Work out the finished part from the listing and answer in its coordinate system (mm). A direction names the side the tool comes from. Coordinates: 2 decimals unless noted, no trailing zeros. Order: outer loops, then holes, each group sorted by start corner. A loop starts at its lowest first (then second) coordinate and runs counter-clockwise, first axis right, second up.
```python
from build123d import *

# Parameters (mm, degrees)
EXTRUDE_1_DEPTH     = 25
EXTRUDE_3_DEPTH     = 4
EXTRUDE_4_DEPTH     = 4
EXTRUDE_5_DEPTH     = 4
EXTRUDE_6_DEPTH     = 4
EXTRUDE_7_DEPTH     = 7
SKETCH_7_W          = 23
SKETCH_7_H          = 20
EXTRUDE_8_DEPTH     = 8.5
SKETCH_8_W          = 16.231712275
SKETCH_8_H          = 15.860541866
EXTRUDE_9_DEPTH     = 3
FILLET_1_R          = 3
FILLET_2_R          = 1
SKETCH_9_R          = 10.42057087
CUT_EXTRUDE_1_DEPTH = 1
SKETCH_10_R         = 10.197555966
CUT_EXTRUDE_2_DEPTH = 1


with BuildPart() as part:
    # ｽｹｯﾁ1 → ﾎﾞｽ - 押し出し1 (new body)
    with BuildSketch(Plane.XY):
        with BuildLine():
            Line((7, 0), (32, 0))
            ThreePointArc((32, 0), (36.949747468, 2.050252532), (39, 7))
            Line((39, 7), (39, 27))
            ThreePointArc((39, 27), (36.949747468, 31.949747468), (32, 34))
            Line((32, 34), (7, 34))
            ThreePointArc((7, 34), (2.050252532, 31.949747468), (0, 27))
            Line((0, 27), (0, 7))
            ThreePointArc((0, 7), (2.050252532, 2.050252532), (7, 0))
        make_face()
    extrude(amount=EXTRUDE_1_DEPTH)

    # ｽｹｯﾁ2 → ﾎﾞｽ - 押し出し3 (add)
    with BuildSketch(Plane(origin=(0, 0, 0), x_dir=(-1, 0, 0), z_dir=(0, 0, -1))):
        with BuildLine():
            Line((-37, 27), (-37, 7))
            ThreePointArc((-37, 7), (-35.535533906, 3.464466094), (-32, 2))
            Line((-32, 2), (-7, 2))
            ThreePointArc((-7, 2), (-3.464466094, 3.464466094), (-2, 7))
            Line((-2, 7), (-2, 27))
            ThreePointArc((-2, 27), (-3.464466094, 30.535533906), (-7, 32))
            Line((-7, 32), (-32, 32))
            ThreePointArc((-32, 32), (-35.535533906, 30.535533906), (-37, 27))
        make_face()
    extrude(amount=EXTRUDE_3_DEPTH)

    # ｽｹｯﾁ3 → ﾎﾞｽ - 押し出し4 (add)
    with BuildSketch(Plane(origin=(0, 0, -4), x_dir=(-1, 0, 0), z_dir=(0, 0, -1))):
        with BuildLine():
            Line((-32, 2.4), (-7, 2.4))
            ThreePointArc((-7, 2.4), (-3.747308807, 3.747308807), (-2.4, 7))
            Line((-2.4, 7), (-2.4, 27))
            ThreePointArc((-2.4, 27), (-3.747308807, 30.252691193), (-7, 31.6))
            Line((-7, 31.6), (-32, 31.6))
            ThreePointArc((-32, 31.6), (-35.252691193, 30.252691193), (-36.6, 27))
            Line((-36.6, 27), (-36.6, 7))
            ThreePointArc((-36.6, 7), (-35.252691193, 3.747308807), (-32, 2.4))
        make_face()
    extrude(amount=EXTRUDE_4_DEPTH)

    # ｽｹｯﾁ4 → ﾎﾞｽ - 押し出し5 (add)
    with BuildSketch(Plane(origin=(0, 0, -8), x_dir=(-1, 0, 0), z_dir=(0, 0, -1))):
        with BuildLine():
            Line((-36.2, 27), (-36.2, 7))
            ThreePointArc((-36.2, 7), (-34.969848481, 4.030151519), (-32, 2.8))
            Line((-32, 2.8), (-7, 2.8))
            ThreePointArc((-7, 2.8), (-4.030151519, 4.030151519), (-2.8, 7))
            Line((-2.8, 7), (-2.8, 27))
            ThreePointArc((-2.8, 27), (-4.030151519, 29.969848481), (-7, 31.2))
            Line((-7, 31.2), (-32, 31.2))
            ThreePointArc((-32, 31.2), (-34.969848481, 29.969848481), (-36.2, 27))
        make_face()
    extrude(amount=EXTRUDE_5_DEPTH)

    # ｽｹｯﾁ5 → ﾎﾞｽ - 押し出し6 (add)
    with BuildSketch(Plane(origin=(0, 0, -12), x_dir=(-1, 0, 0), z_dir=(0, 0, -1))):
        with BuildLine():
            Line((-35.8, 27), (-35.8, 7))
            ThreePointArc((-35.8, 7), (-34.687005769, 4.312994231), (-32, 3.2))
            Line((-32, 3.2), (-7, 3.2))
            ThreePointArc((-7, 3.2), (-4.312994231, 4.312994231), (-3.2, 7))
            Line((-3.2, 7), (-3.2, 27))
            ThreePointArc((-3.2, 27), (-4.312994231, 29.687005769), (-7, 30.8))
            Line((-7, 30.8), (-32, 30.8))
            ThreePointArc((-32, 30.8), (-34.687005769, 29.687005769), (-35.8, 27))
        make_face()
    extrude(amount=EXTRUDE_6_DEPTH)

    # ｽｹｯﾁ6 → ﾎﾞｽ - 押し出し7 (add)
    with BuildSketch(Plane(origin=(0, 0, -16), x_dir=(-1, 0, 0), z_dir=(0, 0, -1))):
        with BuildLine():
            Line((-35.4, 27), (-35.4, 7))
            ThreePointArc((-35.4, 7), (-34.404163056, 4.595836944), (-32, 3.6))
            Line((-32, 3.6), (-7, 3.6))
            ThreePointArc((-7, 3.6), (-4.595836944, 4.595836944), (-3.6, 7))
            Line((-3.6, 7), (-3.6, 27))
            ThreePointArc((-3.6, 27), (-4.595836944, 29.404163056), (-7, 30.4))
            Line((-7, 30.4), (-32, 30.4))
            ThreePointArc((-32, 30.4), (-34.404163056, 29.404163056), (-35.4, 27))
        make_face()
    extrude(amount=EXTRUDE_7_DEPTH)

    # ｽｹｯﾁ7 → ﾎﾞｽ - 押し出し8 (add)
    with BuildSketch(Plane.ZY.offset(-3.6)):
        with Locations((-11.5, 17)):
            Rectangle(SKETCH_7_W, SKETCH_7_H)
    extrude(amount=EXTRUDE_8_DEPTH)

    # ｽｹｯﾁ8 → ﾎﾞｽ - 押し出し9 (add)
    with BuildSketch(Plane(origin=(39, 0, 0), x_dir=(0, 0, -1), z_dir=(1, 0, 0))):
        with Locations((-16.884143863, 17.283223962)):
            Rectangle(SKETCH_8_W, SKETCH_8_H)
    extrude(amount=EXTRUDE_9_DEPTH)

    # ﾌｨﾚｯﾄ1
    fillet_1_edges = [part.edges().sort_by_distance(p)[0] for p in [
        (39, 26.106747447, 25),
        (40.5, 25.213494895, 25),
        (42, 17.283223962, 25),
        (40.5, 9.352953029, 25),
        (39, 8.176476514, 25),
        (36.949747468, 2.050252532, 25),
        (19.5, 0, 25),
        (2.050252532, 2.050252532, 25),
        (0, 17, 25),
        (2.050252532, 31.949747468, 25),
        (19.5, 34, 25),
        (36.949747468, 31.949747468, 25),
    ]]
    fillet(fillet_1_edges, radius=FILLET_1_R)

    # ﾌｨﾚｯﾄ2
    fillet_2_edges = [part.edges().sort_by_distance(p)[0] for p in [
        (34.404163056, 29.404163056, -23),
        (35.4, 17, -23),
        (34.404163056, 4.595836944, -23),
        (19.5, 3.6, -23),
        (4.595836944, 4.595836944, -23),
        (4.595836944, 29.404163056, -23),
        (19.5, 30.4, -23),
        (-0.65, 7, -23),
        (-0.65, 27, -23),
        (-4.9, 17, -23),
    ]]
    fillet(fillet_2_edges, radius=FILLET_2_R)

    # ｽｹｯﾁ9 → ｶｯﾄ - 押し出し1 (cut)
    with BuildSketch(Plane.XY.offset(25)):
        with Locations((19.497752913, 17.033640908)):
            Circle(SKETCH_9_R)
    extrude(amount=-CUT_EXTRUDE_1_DEPTH, mode=Mode.SUBTRACT)

    # ｽｹｯﾁ10 → ｶｯﾄ - 押し出し2 (cut)
    with BuildSketch(Plane(origin=(0, 0, -23), x_dir=(-1, 0, 0), z_dir=(0, 0, -1))):
        with Locations((-19.633872533, 17.026501787)):
            Circle(SKETCH_10_R)
    extrude(amount=-CUT_EXTRUDE_2_DEPTH, mode=Mode.SUBTRACT)


solid = part.part
```
1. For faces 4 (the flat face through (19, 31.6, -6)), 5 (the flat face through (0, 17, 11)), 6 (the cylindrical face through (4.343, 4.284, -13.972)), 7 (the cylindrical face through (4.57, 29.38, -18.96)), determine the directions among +Z, -Z, +X, -X, +Y, -Y from which every point of the face is accessible in a straight line to the end or side of a thin tool.
2. The part is cut by section D-D (z = 9.5). Determine the outline of the cut face in (x, y).
3. The part is cut by section B-B (x = 31). Determine the outline of the cut face in (y, z).
4. The mould has two halves that part along Y. Classify faces 1 (the flat face through (36.2, 17, -10)), 2 (the cylindrical face through (4.284, 29.657, -13.972)), 3 (the flat face through (19, 17, 24)): released by +Y, released by -Y, zero draft, split by the parting line, or undercut.
5. The part is cut by section A-A (z = -9). Determine the outline of the cut face in (x, y).
6. Flat-ended cylindrical pins translate along their axes: pin 1 (4 mm diameter, centred on x = -0.5, z = -15, fed in from -Y); pin 2 (2 mm diameter, centred on x = 25.5, z = -13.5, fed in from +Y); pin 3 (2 mm diameter, centred on x = 17, z = -6.5, fed in from +Y). Find the tip coordinate at first contact, or state that the pin passes through.
7. Consider probe 1 along X at (y, z) = (20.5, 11); probe 2 along Z at (x, y) = (11, 14); probe 3 along X at (y, z) = (17.5, -10). Determine where each line is inside the solid, lowest interval first.
Worked out:
1. face 4: -Z, +X, -X, +Y
1. face 5: +Z, -X, +Y, -Y
1. face 6: -Z, -X, -Y
1. face 7: -Z, -X, +Y
2. outline: (0, 7) arc R7 ccw to (7, 0) - (32, 0) arc R7 ccw to (39, 7) - (39, 9.35) - (42, 9.35) - (42, 25.21) - (39, 25.21) - (39, 27) arc R7 ccw to (32, 34) - (7, 34) arc R7 ccw to (0, 27) - close
3. outline: (0, 0) - (2, 0) - (2, -4) - (2.4, -4) - (2.4, -8) - (2.8, -8) - (2.8, -12) - (3.2, -12) - (3.2, -16) - (3.6, -16) - (3.6, -22) arc R1 ccw to (4.6, -23) - (29.4, -23) arc R1 ccw to (30.4, -22) - (30.4, -16) - (30.8, -16) - (30.8, -12) - (31.2, -12) - (31.2, -8) - (31.6, -8) - (31.6, -4) - (32, -4) - (32, 0) - (34, 0) - (34, 22) arc R3 ccw to (31, 25) - (3, 25) arc R3 ccw to (0, 22) - close
4. face 1: zero draft
4. face 2: released by +Y
4. face 3: undercut
5. outline: (-4.9, 7) - (2.8, 7) arc R4.2 ccw to (7, 2.8) - (32, 2.8) arc R4.2 ccw to (36.2, 7) - (36.2, 27) arc R4.2 ccw to (32, 31.2) - (7, 31.2) arc R4.2 ccw to (2.8, 27) - (-4.9, 27) - close
6. pin 1: stops at y = 7
6. pin 2: stops at y = 30.8
6. pin 3: stops at y = 31.6
7. probe 1: x = 0 to 42
7. probe 2: z = -22 to 24
7. probe 3: x = -4.9 to 36.2
